from build123d import *

# Parameters (mm, degrees)
SKETCH2_R          = 1.6
CUT_EXTRUDE1_DEPTH = 17
SKETCH3_R          = 1.5
CUT_EXTRUDE2_DEPTH = 15


with BuildPart() as part:
    # Sketch1 → Revolve1 (revolve)
    with BuildSketch(Plane.XY):
        Polygon((-14, 0), (-14, 4), (-7.5, 4), (-7.5, 16), (-2, 16), (-2, 0), align=None)
    revolve(axis=Axis((0, 0, 0), (0, -1, 0)))

    # Sketch2 → Cut-Extrude1 (cut, through all)
    with BuildSketch(Plane(origin=(0, 0, 0), x_dir=(1, 0, 0), z_dir=(0, 1, 0))):
        with Locations((0, 10.5)):
            Circle(SKETCH2_R)
        with Locations((9.09326674, -5.25)):
            Circle(SKETCH2_R)
        with Locations((-9.09326674, -5.25)):
            Circle(SKETCH2_R)
    extrude(amount=CUT_EXTRUDE1_DEPTH, mode=Mode.SUBTRACT)

    # Sketch3 → Cut-Extrude2 (cut, through all)
    with BuildSketch(Plane.XY):
        with Locations((0, 8)):
            Circle(SKETCH3_R)
    extrude(amount=CUT_EXTRUDE2_DEPTH, mode=Mode.SUBTRACT)


solid = part.part
Could you check a few things on this model? Use its own coordinates, in mm. A direction names the side the tool comes from. Give positions to 0.01 mm unless a question says otherwise; leave off trailing zeros. Order: outer loops, then holes, each group sorted by start corner. A loop starts at its lowest first (then second) coordinate and runs counter-clockwise, first axis right, second up. Notation, with made-up numbers: (83, 7) - (101, 7) arc R21 ccw to (101, 13) - close; hole circle Ø7 at (65, -28.5). An arc over 180 degrees is marked (long way). One line per item, written item: value. Start each with the question number.
1. Imagine slicing it at A-A on z = 0. List the corners of the cut face in (x, y) for me.
2. For P1, Ø1.5, axis at x = 2, y = 7.5, coming from the -Z side; P2, Ø8, axis at y = 12.5, z = 5, coming from the -X side; P3, Ø8, axis at x = -2, y = 11.5, coming from the +Z side, each with a flat end and sliding along its axis, tell me the tip position at first contact or that it passes through.
3. If I drill on probe 1 along Z at (x, y) = (0, 1.05); probe 2 along Y at (x, z) = (0, 3.5); probe 3 along Y at (x, z) = (9, 9), over which ranges is the centre line in solid material (lowest first)?
4. Imagine slicing it at B-B on x = 0. List the corners of the cut face in (y, z) for me.
5. Thinking about a two-plate mould opening in Y: for faces 1 (the face through (-0.325, 6.536, 4.37)), 2 (the face through (-6, 4, 6)), 3 (the face through (-12.932, 2.028, 5.362)), which applies, +Y half, -Y half, draft (parallel to the pull), parting line (faces both ways), or undercut?
6. For faces 4 (the face through (7.493, 10.084, -0.33)), 5 (the face through (-0.35, 1.97, -8.94)), which set-ups out of +Z, -Z, +X, -X, +Y, -Y let a thin tool reach every point of the face, with its end or its side?
7. Imagine slicing it at D-D on y = 4.5. List the corners of the cut face in (x, z) for me, plus the area to 3 significant figures.
8. Imagine slicing it at C-C on z = 5.25. List the corners of the cut face in (x, y) for me.
Values:
1. outline: (-14, 0) - (-2, 0) - (-2, 16) - (-7.5, 16) - (-7.5, 4) - (-14, 4) - close; (2, 0) - (14, 0) - (14, 4) - (7.5, 4) - (7.5, 16) - (2, 16) - close
2. P1: z = -7.4
2. P2: x = -7.43
2. P3: z = 7.5
3. probe 1: -14 to -12.1, -8.9 to -2, 2 to 14
3. probe 2: 0 to 6.5, 9.5 to 16
3. probe 3: 0 to 4
4. outline: (0, -14) - (4, -14) - (4, -12.1) - (0, -12.1) - close; (0, -8.9) - (4, -8.9) - (4, -7.5) - (16, -7.5) - (16, -2) - (0, -2) - close; (0, 2) - (6.5, 2) - (6.5, 7.5) - (4, 7.5) - (4, 14) - (0, 14) - close; (9.5, 2) - (16, 2) - (16, 7.5) - (9.5, 7.5) - close
5. face 1: undercut
5. face 2: +Y half
5. face 3: draft
6. face 4: +Y
6. face 5: +Y, -Y
7. outline: circle Ø15 at (0, 0); hole circle Ø4 at (0, 0)
7. area: 164 mm²
8. outline: (-12.98, 0) - (-10.69, 0) - (-10.69, 4) - (-12.98, 4) - close; (-7.49, 0) - (7.49, 0) - (7.49, 4) - (5.36, 4) - (5.36, 16) - (-5.36, 16) - (-5.36, 4) - (-7.49, 4) - close; (10.69, 0) - (12.98, 0) - (12.98, 4) - (10.69, 4) - close; hole circle Ø3 at (0, 8)
